The model under review builds one solid part; all positions refer to its coordinate system, in mm. A direction names the side the tool comes from. Coordinates: 2 decimals unless noted, no trailing zeros. Loops run counter-clockwise (first coordinate to the right, second up) from the corner with the lowest first, then second, coordinate; pieces in that order, holes last. Notation, with made-up numbers: (34, 78) - (53, 78) arc R19 cw to (53, 103) - close; hole circle Ø5 at (-0.5, 36.25). An arc over 180 degrees is marked (long way). Use a Markdown table: item, result. Add a question column.
1) Add section B-B, the plane y = 10.25. Give the boundary of the cut face in (x, z), and give its area (3 significant figures).
2) Add section A-A, the plane x = -132.5. Give the boundary of the cut face in (y, z), and give its area (3 significant figures).
3) For faces 1 (the flat face through (3, 3.2, -2)), 2 (the flat face through (250, 3, 5)), list the 3-axis set-ups (+Z, -Z, +X, -X, +Y, -Y) from which the entire face can be reached by the end or side of a thin tool; tool diameter is ignored.
4) To check wall thickness, follow L1, parallel to Z at x = 116, y = 12.5; L2, parallel to Y at x = -102.5, z = 2.75; L3, parallel to Y at x = -89, z = 10.75. State the ranges of each line that lie inside material, in increasing order. Write a range as [from, to].
5) Add section C-C, the plane z = -3.5. Give the boundary of the cut face in (x, y), and give its area (3 significant figures).
6) Clearance check with flat-ended pins moving along their axes: pin 1 (6 mm diameter, centred on x = 46, z = 0.5, fed in from +Y); pin 2 (2 mm diameter, centred on x = -112, y = 11.5, fed in from -Z). State where each tip first meets the part, or that it passes through.
Autodesk Inventor part; units mm, degrees
ref_plane "YZ Plane" through (0, 0, 0) normal (1, 0, 0) x (0, 1, 0)
ref_plane "XZ Plane" through (0, 0, 0) normal (0, 1, 0) x (-1, 0, 0)
ref_plane "XY Plane" through (0, 0, 0) normal (0, 0, 1) x (1, 0, 0)
sketch "Sketch1" plane through (0, 0, 0) normal (0, 1, 0) x (-1, 0, 0)
  line L0 (-250, 12.7) -> (250, 12.7)
  line L1 (250, 12.7) -> (250, -12.7)
  line L2 (250, -12.7) -> (-250, -12.7)
  line L3 (-250, -12.7) -> (-250, 12.7)
  line L4 (-250, 12.7) -> (250, -12.7) construction
  line L5 (250, 12.7) -> (-250, -12.7) construction
  point P0 (0, 0)
  dimension "d0" = 500
  dimension "d1" = 25.4
extrude "Plate1" add sketch "Sketch1" along normal blind 3.2
sketch "Sketch2" plane through (250, 0, 9.5) normal (0, 0, 1) x (1, 0, 0)
  line L0 (-500, 0) -> (0, 0)
  line L1 (0, 0) -> (0, 22)
  line L2 (0, 22) -> (-500, 22)
  line L3 (-500, 22) -> (-500, 0)
edge flange "Flange1" height 22 angle 90 thickness 3.2 bend radius 1.516 thickness toward (0, 0, 1) relief tear relief width 3.2 relief depth 1.6 edges at (0, 3.2, 12.7) wall of the first edge with corners at (-250, 0, 9.5) (250, 0, 9.5) (250, 22, 9.5) (-250, 22, 9.5)
bend "Bend1"
corner "Corner1"
equation "\"d2\" = Thickness"
equation "\"d3\" = BendReliefWidth"
equation "\"d4\" = BendReliefDepth"
equation "\"d5\" = MinimumRemnant"
equation "\"d6\" = TransitionRadius"
equation "\"d9\" = BendRadius"
equation "\"d10\" = CornerReliefSize"
equation "\"d11\" = GapSize"
equation "\"d12\" = JacobiRadiusSize"
equation "\"BendReliefWidth\" = Thickness"
equation "\"BendReliefDepth\" = 0.5 * Thickness"
equation "\"CornerReliefSize\" = 4 * Thickness"
equation "\"MinimumRemnant\" = 2 * Thickness"
equation "\"TransitionRadius\" = BendRadius"
equation "\"JacobiRadiusSize\" = BendRadius"
equation "\"GapSize\" = Thickness"
properties part number "SP33V1 Tope Base"
From the geometry:
| question | item | result |
|---|---|---|
| 1 | outline | (-250, 9.5) - (250, 9.5) - (250, 12.7) - (-250, 12.7) - close |
| 1 | area | 1,600 mm^2 |
| 2 | outline | (0, -12.7) - (3.2, -12.7) - (3.2, 7.98) arc R1.52 cw to (4.72, 9.5) - (22, 9.5) - (22, 12.7) - (4.72, 12.7) arc R4.72 ccw to (0, 7.98) - close |
| 2 | area | 137 mm^2 |
| 3 | face 1 | -Z, +X, -X, +Y |
| 3 | face 2 | +Z, -Z, +X, +Y, -Y |
| 4 | L1 | z = [9.5, 12.7] |
| 4 | L2 | y = [0, 3.2] |
| 4 | L3 | y = [0.9, 22] |
| 5 | outline | (-250, 0) - (250, 0) - (250, 3.2) - (-250, 3.2) - close |
| 5 | area | 1,600 mm^2 |
| 6 | pin 1 | stops at y = 3.2 |
| 6 | pin 2 | stops at z = 9.5 |
